from build123d import *

# Parameters (mm, degrees)
SKETCH2_W           = 40
SKETCH2_H           = 60
SKETCH2_R           = 1.75
SKETCH2_W_2         = 22
SKETCH2_H_2         = 42
BOSS_EXTRUDE1_DEPTH = 10
BOSS_EXTRUDE3_DEPTH = 10
LPATTERN2_COUNT     = 2
LPATTERN2_PITCH     = 30
SKETCH5_R           = 1.25
CUT_EXTRUDE1_DEPTH  = 12


with BuildPart() as part:
    # Sketch2 → Boss-Extrude1 (new body)
    with BuildSketch(Plane.XY):
        Rectangle(SKETCH2_W, SKETCH2_H)
        with Locations((-5, 24.75)):
            Circle(SKETCH2_R, mode=Mode.SUBTRACT)
        with Locations((5, 24.75)):
            Circle(SKETCH2_R, mode=Mode.SUBTRACT)
        with Locations((-5, -24.75)):
            Circle(SKETCH2_R, mode=Mode.SUBTRACT)
        with Locations((5, -24.75)):
            Circle(SKETCH2_R, mode=Mode.SUBTRACT)
        Rectangle(SKETCH2_W_2, SKETCH2_H_2, mode=Mode.SUBTRACT)
    extrude(amount=BOSS_EXTRUDE1_DEPTH)

    # Sketch4 → Boss-Extrude3 (add)
    with BuildSketch(Plane(origin=(20, 0, 0), x_dir=(0, 0, -1), z_dir=(1, 0, 0))):
        Polygon((0, -30), (25, -30), (0, 30), (-10, 30), (-10, -30), align=None)
    boss_extrude3 = extrude(amount=-BOSS_EXTRUDE3_DEPTH)

    # LPattern2: Boss-Extrude3 ×2
    with Locations(*[(-i * LPATTERN2_PITCH, 0, 0) for i in range(1, LPATTERN2_COUNT)]):
        add(boss_extrude3)

    # Sketch5 → Cut-Extrude1 (cut)
    with BuildSketch(Plane.XZ.offset(30)):
        with Locations((-16, -16.7433949)):
            Circle(SKETCH5_R)
        with Locations((-16, 3.2566051)):
            Circle(SKETCH5_R)
        with Locations((-16, -6.7433949)):
            Circle(SKETCH5_R)
        with Locations(Location((16, -16.7433949, 0), (0, 0, 180))):
            Circle(SKETCH5_R)
        with Locations(Location((16, -6.7433949, 0), (0, 0, 180))):
            Circle(SKETCH5_R)
        with Locations(Location((16, 3.2566051, 0), (0, 0, 180))):
            Circle(SKETCH5_R)
    extrude(amount=-CUT_EXTRUDE1_DEPTH, mode=Mode.SUBTRACT)


solid = part.part
Here's how the part is built. I have some questions about the finished solid (model axes, mm). A direction names the side the tool comes from. Coordinates: 2 decimals unless noted, no trailing zeros. Loops run counter-clockwise (first coordinate to the right, second up) from the corner with the lowest first, then second, coordinate; pieces in that order, holes last.
1. If we mould it in two halves opening along Y, with no side actions, what happens to faces 1 (the cylindrical face through (-5.228, 26.485, 4.93)), 2 (the flat face through (20, -6, -3)), 3 (the flat face through (0, -30, 1))? For each: pulls with the +Y half, pulls with the -Y half, needs draft (parallel to the pull), parting line crosses it, or undercut.
2. For P1, Ø5.5, axis at x = 5, y = 24.75, coming from the -Z side; P2, Ø2, axis at x = -13, y = -5, coming from the -Z side; P3, Ø1.5, axis at x = 13, z = -9.5, coming from the +Y side, each with a flat end and sliding along its axis, tell me the tip position at first contact or that it passes through.
3. Imagine slicing it at D-D, the plane x = 1. Please give me the cut outline in (y, z).
4. For faces 4 (the flat face through (0, 26, 0)), 5 (the flat face through (-20, -6, -3)), 6 (the flat face through (16, -18, 3)), 7 (the flat face through (0, 21, 5)), 8 (the flat face through (0, 30, 5)), which set-ups out of +Z, -Z, +X, -X, +Y, -Y let a thin tool reach every point of the face, with its end or its side?
5. Imagine slicing it at B-B, the plane x = -5. Please give me the cut outline in (y, z).
6. Imagine slicing it at A-A, the plane z = -21. Please give me the cut outline in (x, y).
7. I need wall thicknesses on L1, parallel to X at y = -6, z = -9; L2, parallel to Y at x = -5, z = 4.5; L3, parallel to Z at x = -16, y = -22.75. Which ranges of each line are inside material? Lowest first, please.
8. Imagine slicing it at C-C, the plane y = -24.75. Count the separate pieces of the cut face and the enclosed holes in it, and give its area (3 significant figures).
Taken from the geometry:
1. face 1: undercut
1. face 2: needs draft
1. face 3: pulls with the -Y half
2. P1: stops at z = 0
2. P2: stops at z = -15
2. P3: stops at y = 9
3. outline: (-30, 0) - (-21, 0) - (-21, 10) - (-30, 10) - close; (21, 0) - (30, 0) - (30, 10) - (21, 10) - close
4. face 4: -Z, +Y, -Y
4. face 5: +Z, -Z, -X, +Y, -Y
4. face 6: -Y
4. face 7: +Z, -Z
4. face 8: +Z, -Z, +X, -X, +Y
5. outline: (-30, 0) - (-26.5, 0) - (-26.5, 10) - (-30, 10) - close; (-23, 0) - (-21, 0) - (-21, 10) - (-23, 10) - close; (21, 0) - (23, 0) - (23, 10) - (21, 10) - close; (26.5, 0) - (30, 0) - (30, 10) - (26.5, 10) - close
6. outline: (-20, -30) - (-10, -30) - (-10, -20.4) - (-20, -20.4) - close; (10, -30) - (20, -30) - (20, -20.4) - (10, -20.4) - close
7. L1: x = -20 to -10, 10 to 20
7. L2: y = -30 to -26.5, -23 to -21, 21 to 23, 26.5 to 30
7. L3: z = -21.98 to -17.99, -15.49 to -7.99, -5.49 to 2.01, 4.51 to 10
8. separate pieces: 3
8. enclosed holes: 6
8. area: 757 mm2
